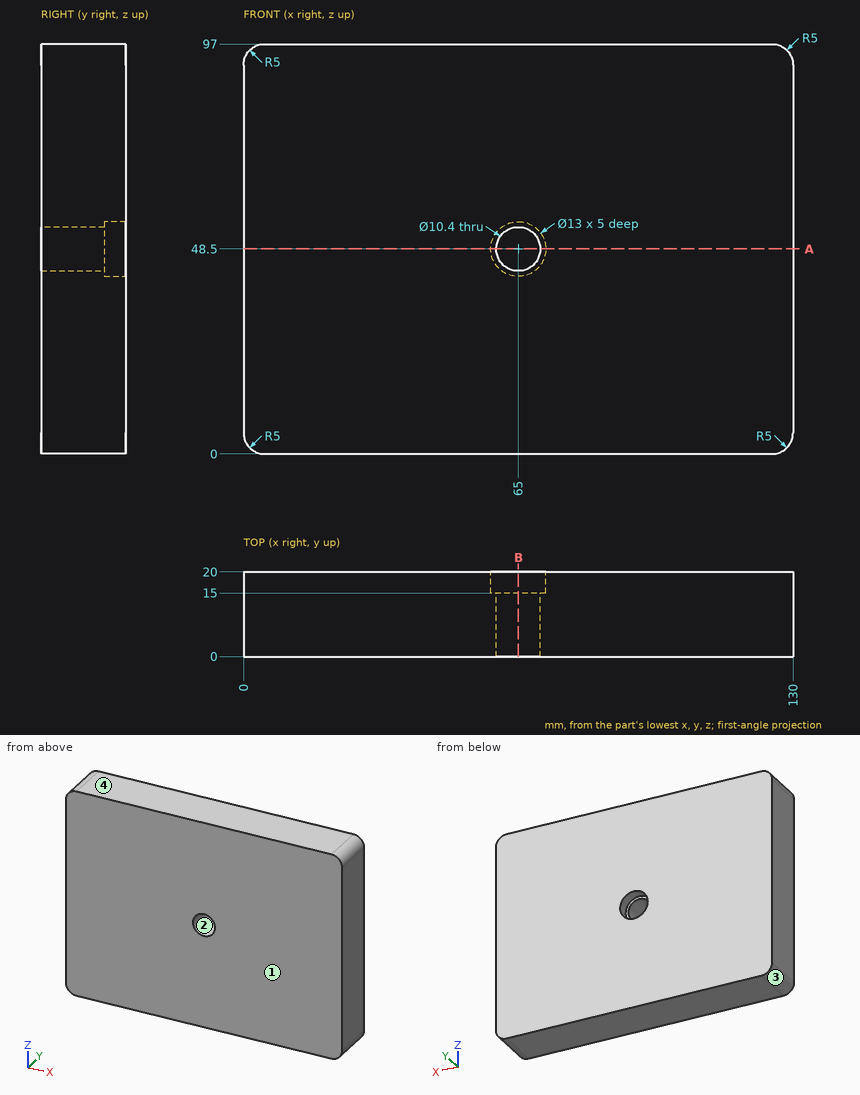
Design review of the part shown in the three views and the two pictorial views. Dimensions are in mm from the part's minimum x, y and z. Round coordinates to 2 decimals unless told otherwise and drop trailing zeros. Loops run counter-clockwise (first coordinate to the right, second up) from the corner with the lowest first, then second, coordinate; pieces in that order, holes last.
Q1. Mouldability with a two-part tool opening along Z and no side actions: class the marked faces 1, 2, 3 and 4 as +Z half, -Z half, draft (parallel to the pull), parting line (faces both ways), or undercut.
Result sheet:
face 1: draft
face 2: undercut
face 3: -Z half
face 4: +Z half
Q2. Add section B-B on x = 65. Write out the cut boundary in (y, z).
Result sheet:
outline: (0, 0) - (20, 0) - (20, 42) - (15, 42) - (15, 43.3) - (0, 43.3) - close; (0, 53.7) - (15, 53.7) - (15, 55) - (20, 55) - (20, 97) - (0, 97) - close
Q3. Add section A-A on z = 48.5. Write out the cut boundary in (x, y), plus the area to 3 significant figures.
Result sheet:
outline: (0, 0) - (59.8, 0) - (59.8, 15) - (58.5, 15) - (58.5, 20) - (0, 20) - close; (70.2, 0) - (130, 0) - (130, 20) - (71.5, 20) - (71.5, 15) - (70.2, 15) - close
area: 2,380 mm2
Q4. To check wall thickness, follow line 1 along X through (y, z) = (4.5, 48.5); line 2 along X through (y, z) = (18.9, 48.5). State the ranges of each line that lie inside material, in increasing order.
Result sheet:
line 1: x = 0 to 59.8, 70.2 to 130
line 2: x = 0 to 58.5, 71.5 to 130
